```python
from build123d import *

# Parameters (mm, degrees)
BOX_W                       = 2
BOX_H                       = 2
BOX_DEPTH                   = 2
CYLINDER_R                  = 1
CYLINDER_DEPTH              = 7
ARRAY_COUNT                 = 8
ARRAY_ANGLE                 = -66.734026
ARRAY_PLACEMENT_ANGLE       = 22.8
TUBE001_R                   = 26.5
TUBE001_R_2                 = 22
TUBE001_DEPTH               = 5
CYLINDER003_W               = 27
CYLINDER003_H               = 10
CYLINDER003_ANGLE           = 81.734026
CYLINDER003_PLACEMENT_ANGLE = 43
COMMON001_PLACEMENT_ANGLE   = 4


with BuildPart() as cube:
    # Box → Box (new body)
    with BuildSketch(Plane(origin=(-1, 21, 0), x_dir=(1, 0, 0), z_dir=(0, 0, 1))):
        with Locations((1, 1)):
            Rectangle(BOX_W, BOX_H)
    extrude(amount=BOX_DEPTH)


with BuildPart() as bodyside_contacts:
    # Cylinder → Cylinder (new body)
    with BuildSketch(Plane(origin=(0, 29, 1), x_dir=(1, 0, 0), z_dir=(0, -1, 0))):
        Circle(CYLINDER_R)
    extrude(amount=CYLINDER_DEPTH)

    # Fusion: union Cube
    add(cube.part)

    # Array: BodySide_Contacts ×8 about axis
    array_axis = Axis((0, 0, 0), (0, 0, 1))


with BuildPart() as bodyside_contacts_1:
    add(bodyside_contacts.part)
    for i in range(1, ARRAY_COUNT):
        add(bodyside_contacts.part.rotate(array_axis, i * ARRAY_ANGLE / (ARRAY_COUNT - 1)))


with BuildPart() as bodyside_contacts_2:
    # Array placement: moved
    add(bodyside_contacts_1.part.rotate(Axis((0, 0, 0), (0, 0, 1)), ARRAY_PLACEMENT_ANGLE))


with BuildPart() as tube001:
    # Tube001 → Tube001 (new body)
    with BuildSketch(Plane.XY.offset(-1.5)):
        Circle(TUBE001_R)
        Circle(TUBE001_R_2, mode=Mode.SUBTRACT)
    extrude(amount=TUBE001_DEPTH)


with BuildPart() as cut001:
    # Cylinder003 → Cylinder003 (revolve)
    with BuildSketch(Plane.XZ):
        with Locations((13.5, 5)):
            Rectangle(CYLINDER003_W, CYLINDER003_H)
    revolve(axis=Axis((0, 0, 0), (0, 0, 1)), revolution_arc=CYLINDER003_ANGLE)


with BuildPart() as cut001_1:
    # Cylinder003 placement: moved
    add(cut001.part.moved(Location((0, 0, -3))).rotate(Axis((0, 0, -3), (0, 0, 1)), CYLINDER003_PLACEMENT_ANGLE))

    # Common001: intersect Tube001
    add(tube001.part, mode=Mode.INTERSECT)


with BuildPart() as cut001_2:
    # Common001 placement: moved
    add(cut001_1.part.rotate(Axis((0, 0, 0), (0, 0, -1)), COMMON001_PLACEMENT_ANGLE))

    # Cut001: cut BodySide_Contacts
    add(bodyside_contacts_2.part, mode=Mode.SUBTRACT)


solid = cut001_2.part
```
Build history of the part. All positions in model axes, mm. A direction names the side the tool comes from. Give positions to 0.01 mm unless a question says otherwise; leave off trailing zeros. Loops run counter-clockwise (first coordinate to the right, second up) from the corner with the lowest first, then second, coordinate; pieces in that order, holes last.
1) Two-plate mould, pull along X, no slides. Class faces 1 (the face through (13.527, 17.985, 0.986)), 2 (the face through (4.92, 26.04, 0.96)), 3 (the face through (3, 22, 3.5)), 4 (the face through (8.547, 20.818, 0.986)): released by +X, released by -X, zero draft, split by the parting line, or undercut.
Values follow:
face 1: released by -X
face 2: split by the parting line
face 3: zero draft
face 4: undercut
2) Band-saw the part on A-A on z = -0.9. List the corners of the cut face in (x, y), then the cut area to 3 significant figures.
Values follow:
outline: (-13.54, 22.78) - (-11.24, 18.91) arc R22 cw to (17.1, 13.85) - (20.59, 16.68) arc R26.5 ccw to start
area: 156 mm2
3) Probe line 1 along Z through (x, y) = (2.5, 23.5); line 2 along Y through (x, z) = (16.5, 0.2); line 3 along X through (y, z) = (18, 0.85). List the from-to ranges inside material, lowest first.
Values follow:
line 1: z = -1.5 to 0.01, 1.99 to 3.5
line 2: y = 14.55 to 15.68, 16.04 to 16.26, 17.99 to 20.74
line 3: x = 13.54 to 15.97, 18.72 to 19.45
4) 3-axis set-ups, long thin cutter, end or side, ignore diameter. For faces 5 (the face through (12.7, 18.6, 2)), 6 (the face through (4.087, 21.617, 0.965)), 7 (the face through (-7.79, 21.11, 0.99)): which of +Z, -Z, +X, -X, +Y, -Y reach the whole face in a straight line?
Values follow:
face 5: none
face 6: +Z, -Z, -Y
face 7: -Y
5) Drop flat-ended pins along their axis: P1, Ø2, axis at y = 24.5, z = -0.5, coming from the -X side; P2, Ø3, axis at y = 17.5, z = 2, coming from the +X side; P3, Ø1, axis at y = 22, z = 1, coming from the +X side. Give the stop position or say it passes through.
Values follow:
P1: stops at x = -12.25
P2: stops at x = 20.59
P3: stops at x = 14.18
